Here's how the part is built. I have some questions about the finished solid (model axes, mm). Face numbers are marked on the shaded views. A direction names the side the tool comes from. Round coordinates to 2 decimals unless told otherwise and drop trailing zeros. Write each loop counter-clockwise with the first axis right and the second up, starting at its lowest first coordinate (ties: lowest second). Pieces come first, ordered by that corner, then holes. Notation, with made-up numbers: (20.5, 10.25) - (71.5, 10.25) arc R30 ccw to (71.5, 42.25) - close; hole circle Ø11 at (56.5, 14). An arc over 180 degrees is marked (long way). Write item = value, one per line. Start each with the question number.
Item 1: Which directions (+Z, -Z, +X, -X, +Y, -Y) give clear straight access to the entire face, cutting with the end or side of a thin tool? Please do the marked faces 1, 2 and 3.
Item 2: If we section it at A-A (y = 1.5): Please give me the cut outline in (x, z).
Item 3: If I drill on line 1 along X through (y, z) = (11, 11.5); line 2 along X through (y, z) = (2.5, 10); line 3 along Y through (x, z) = (-19, 4), over which ranges is the centre line in solid material (lowest first)? Write a range as [from, to].
Item 4: If we section it at C-C (y = 11): Please give me the cut outline in (x, z), and give its area (3 significant figures).
Item 5: Thinking about a two-plate mould opening in Z: for the marked faces 4, 5, 6 and 7, which applies, pulls with the +Z half, pulls with the -Z half, needs draft (parallel to the pull), parting line crosses it, or undercut?
Item 6: If we section it at D-D (z = -9.5): Please give me the cut outline in (x, y), and give its area (3 significant figures).
Item 7: For P1, Ø3.5, axis at x = -17.32, z = 10, coming from the -Y side; P2, Ø6.5, axis at x = 0, z = -20, coming from the -Y side; P3, Ø1, axis at x = 17.5, y = 9.5, coming from the -Z side; P4, Ø2.5, axis at x = -17, y = 10, coming from the -Z side, each with a flat end and sliding along its axis, tell me the tip position at first contact or that it passes through.
Item 8: If we section it at B-B (x = -1): Please give me the cut outline in (y, z).
```python
from build123d import *

# Parameters (mm, degrees)
ESQUISSE1_R             = 11.9
ESQUISSE1_R_2           = 2
BOSS_EXTRU_1_DEPTH      = 12
ENL_V_MAT_EXTRU_1_DEPTH = 5
SKETCH1_R               = 11.9
BOSS_EXTRUDE1_DEPTH     = 2
BOSS_EXTRUDE2_START     = 1.5
SKETCH2_R               = 15.5
SKETCH2_R_2             = 11.9
BOSS_EXTRUDE2_DEPTH     = 1.5
BOSS_EXTRUDE3_DEPTH     = 0.1


with BuildPart() as part:
    # Esquisse1 → Boss.-Extru.1 (new body)
    with BuildSketch(Plane(origin=(0, 0, 0), x_dir=(1, 0, 0), z_dir=(0, 1, 0))):
        with BuildLine():
            Line((-6.495190528, 23.75), (-23.815698604, -6.25))
            ThreePointArc((-23.815698604, -6.25), (-23.815698604, -13.75), (-17.320508076, -17.5))
            Line((-17.320508076, -17.5), (17.320508076, -17.5))
            ThreePointArc((17.320508076, -17.5), (23.815698604, -13.75), (23.815698604, -6.25))
            Line((23.815698604, -6.25), (6.495190528, 23.75))
            ThreePointArc((6.495190528, 23.75), (0, 27.5), (-6.495190528, 23.75))
        make_face()
        with Locations(Location((0, 0, 0), (0, 0, 270))):
            Circle(ESQUISSE1_R, mode=Mode.SUBTRACT)
        with Locations(Location((-17.320508076, -10, 0), (0, 0, 270))):
            Circle(ESQUISSE1_R_2, mode=Mode.SUBTRACT)
        with Locations(Location((0, 20, 0), (0, 0, 270))):
            Circle(ESQUISSE1_R_2, mode=Mode.SUBTRACT)
        with Locations(Location((17.320508076, -10, 0), (0, 0, 270))):
            Circle(ESQUISSE1_R_2, mode=Mode.SUBTRACT)
    extrude(amount=BOSS_EXTRU_1_DEPTH)

    # Esquisse2 → Enlèv. mat.-Extru.1 (cut)
    with BuildSketch(Plane(origin=(0, 12, 0), x_dir=(1, 0, 0), z_dir=(0, 1, 0))):
        Polygon((-18.908221316, -7.25), (-20.495934556, -10), (-18.908221316, -12.75), (-15.732794835, -12.75), (-14.145081595, -10), (-15.732794835, -7.25), align=None)
        Polygon((-1.58771324, 22.75), (-3.175426481, 20), (-1.58771324, 17.25), (1.58771324, 17.25), (3.175426481, 20), (1.58771324, 22.75), align=None)
        Polygon((18.908221316, -7.25), (15.732794835, -7.25), (14.145081595, -10), (15.732794835, -12.75), (18.908221316, -12.75), (20.495934556, -10), align=None)
    extrude(amount=-ENL_V_MAT_EXTRU_1_DEPTH, mode=Mode.SUBTRACT)

    # Sketch2 → Boss-Extrude2 (add)
    with BuildSketch(Plane.XZ.offset(BOSS_EXTRUDE2_START)):
        with Locations(Location((0, 0, 0), (0, 0, 90))):
            Circle(SKETCH2_R)
        with Locations(Location((0, 0, 0), (0, 0, 90))):
            Circle(SKETCH2_R_2, mode=Mode.SUBTRACT)
    extrude(amount=-BOSS_EXTRUDE2_DEPTH)



with BuildPart() as body_2:
    # Sketch1 → Boss-Extrude1 (new body)
    with BuildSketch(Plane(origin=(0, 12, 0), x_dir=(1, 0, 0), z_dir=(0, 1, 0))):
        with Locations(Location((0, 0, 0), (0, 0, 270))):
            Circle(SKETCH1_R)
    extrude(amount=-BOSS_EXTRUDE1_DEPTH)


with BuildPart() as part_1:
    add(part.part)

    add(body_2.part)  # Boss-Extrude3 merges body 2
    # Sketch3 → Boss-Extrude3 (add)
    with BuildSketch(Plane(origin=(0, 12, 0), x_dir=(1, 0, 0), z_dir=(0, 1, 0))):
        with BuildLine():
            Line((-6.495190528, 23.75), (-23.815698604, -6.25))
            ThreePointArc((-23.815698604, -6.25), (-23.815698604, -13.75), (-17.320508076, -17.5))
            Line((-17.320508076, -17.5), (17.320508076, -17.5))
            ThreePointArc((17.320508076, -17.5), (23.815698604, -13.75), (23.815698604, -6.25))
            Line((23.815698604, -6.25), (6.495190528, 23.75))
            ThreePointArc((6.495190528, 23.75), (0, 27.5), (-6.495190528, 23.75))
        make_face()
        Polygon((-1.58771324, 22.75), (-3.175426481, 20), (-1.58771324, 17.25), (1.58771324, 17.25), (3.175426481, 20), (1.58771324, 22.75), align=None, mode=Mode.SUBTRACT)
        Polygon((18.908221316, -12.75), (20.495934556, -10), (18.908221316, -7.25), (15.732794835, -7.25), (14.145081595, -10), (15.732794835, -12.75), align=None, mode=Mode.SUBTRACT)
        Polygon((-18.908221316, -7.25), (-20.495934556, -10), (-18.908221316, -12.75), (-15.732794835, -12.75), (-14.145081595, -10), (-15.732794835, -7.25), align=None, mode=Mode.SUBTRACT)
    extrude(amount=BOSS_EXTRUDE3_DEPTH)


solid = part_1.part
```
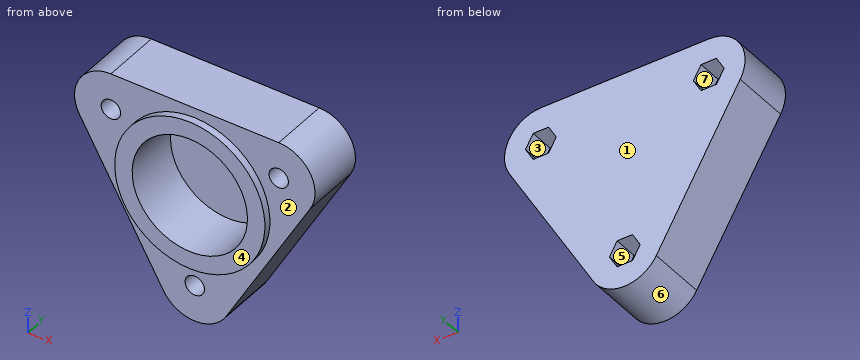
Reply:
q1.face_1 = +Z, -Z, +X, -X, +Y
q1.face_2 = -Y
q1.face_3 = +Y
q2.outline = (-23.82, 6.25) - (-6.5, -23.75) arc R7.5 ccw to (6.5, -23.75) - (23.82, 6.25) arc R7.5 ccw to (17.32, 17.5) - (-17.32, 17.5) arc R7.5 ccw to start; hole circle Ø4 at (-17.32, 10); hole circle Ø23.8 at (0, 0); hole circle Ø4 at (0, -20); hole circle Ø4 at (17.32, 10)
q3.line_1 = [-24.67, -19.63], [-15.01, 15.01], [19.63, 24.67]
q3.line_2 = [-24.82, -19.32], [-15.32, -6.45], [6.45, 15.32], [19.32, 24.82]
q3.line_3 = [0, 12.1]
q4.outline = (-23.82, 6.25) - (-6.5, -23.75) arc R7.5 ccw to (6.5, -23.75) - (23.82, 6.25) arc R7.5 ccw to (17.32, 17.5) - (-17.32, 17.5) arc R7.5 ccw to start; hole (-20.5, 10) - (-18.91, 7.25) - (-15.73, 7.25) - (-14.15, 10) - (-15.73, 12.75) - (-18.91, 12.75) - close; hole (-3.18, -20) - (-1.59, -22.75) - (1.59, -22.75) - (3.18, -20) - (1.59, -17.25) - (-1.59, -17.25) - close; hole (14.15, 10) - (15.73, 7.25) - (18.91, 7.25) - (20.5, 10) - (18.91, 12.75) - (15.73, 12.75) - close
q4.area = 1,400 mm2
q5.face_4 = needs draft
q5.face_5 = undercut
q5.face_6 = pulls with the -Z half
q5.face_7 = undercut
q6.outline = (-14.72, 0) - (-12.25, 0) - (-12.25, -1.5) - (-7.17, -1.5) - (-7.17, 10) - (7.17, 10) - (7.17, -1.5) - (12.25, -1.5) - (12.25, 0) - (14.72, 0) - (14.72, 12.1) - (-14.72, 12.1) - close
q6.area = 228 mm2
q7.P1 = through
q7.P2 = 0
q7.P3 = -5.56
q7.P4 = -7.72
q8.outline = (-1.5, -15.47) - (0, -15.47) - (0, -18.27) - (7, -18.27) - (7, -17.25) - (12.1, -17.25) - (12.1, 17.5) - (0, 17.5) - (0, 15.47) - (-1.5, 15.47) - (-1.5, 11.86) - (10, 11.86) - (10, -11.86) - (-1.5, -11.86) - close; (0, -27.43) - (12.1, -27.43) - (12.1, -22.75) - (7, -22.75) - (7, -21.73) - (0, -21.73) - close
